Model file for the job. Use its own axes, mm. A direction names the side the tool comes from. Round coordinates to 2 decimals unless told otherwise and drop trailing zeros. Order: outer loops, then holes, each group sorted by start corner. A loop starts at its lowest first (then second) coordinate and runs counter-clockwise, first axis right, second up. Notation, with made-up numbers: (81.25, 52.5) -> (120.25, 52.5) arc R29 ccw to (120.25, 91.5) -> close; hole circle Ø9 at (25.5, 11.5). An arc over 180 degrees is marked (long way). Use CSV: the item, a comma, the result in double quotes.
```python
from build123d import *

# Parameters (mm, degrees)
PAD002_DEPTH             = 2.7
CYLINDER_R               = 2.95
CYLINDER_DEPTH           = 7
CYLINDER001_R            = 1.7
CYLINDER001_DEPTH        = 30
CLONE118_PLACEMENT_ANGLE = 180
BOX250_W                 = 10
BOX250_H                 = 10
BOX250_DEPTH             = 20


with BuildPart() as clone_of_m3nuthousing009:
    # Sketch003 → Pad002 (new body)
    with BuildSketch(Plane.XY):
        Polygon((0, 0), (1.674316, 2.9), (21.674316, 2.9), (21.674316, -2.9), (1.674316, -2.9), align=None)
    extrude(amount=PAD002_DEPTH)


with BuildPart() as clone_of_m3nuthousing009_1:
    # Clone119 placement: moved
    add(clone_of_m3nuthousing009.part.moved(Location((1.5, 5, 14))))


with BuildPart() as m3bolthead:
    # Cylinder → Cylinder (new body)
    with BuildSketch(Plane.XY):
        Circle(CYLINDER_R)
    extrude(amount=CYLINDER_DEPTH)


with BuildPart() as fusion051:
    # Cylinder001 → Cylinder001 (new body)
    with BuildSketch(Plane.XY.offset(6)):
        Circle(CYLINDER001_R)
    extrude(amount=CYLINDER001_DEPTH)

    # Fusion: union M3BoltHead
    add(m3bolthead.part)


with BuildPart() as fusion051_1:
    # Clone118 placement: moved
    add(fusion051.part.moved(Location((5, 5, 40))).rotate(Axis((5, 5, 40), (1, 0, 0)), CLONE118_PLACEMENT_ANGLE))

    # Fusion051: union Clone of M3NutHousing009
    add(clone_of_m3nuthousing009_1.part)


with BuildPart() as obj1:
    # Box250 → Box250 (new body)
    with BuildSketch(Plane.XY):
        with Locations((5, 5)):
            Rectangle(BOX250_W, BOX250_H)
    extrude(amount=BOX250_DEPTH)

    # Cut040: cut Fusion051
    add(fusion051_1.part, mode=Mode.SUBTRACT)


solid = obj1.part
```
Q1. Pin check, flat tip, straight feed: pin 1 (3 mm diameter, centred on x = 5, y = 5, fed in from +Z). Stop position of the tip, or through.
From the geometry:
pin 1,"stops at z = 4"
Q2. Mould opens along Y. For faces 1 (the cylindrical face through (4.63, 6.66, 18.37)), 2 (the flat face through (5, 10, 10)), 3 (the flat face through (5, 5, 0)) say: +Y half, -Y half, draft (parallel to the pull), parting line (faces both ways), or undercut.
From the geometry:
face 1,"undercut"
face 2,"+Y half"
face 3,"draft"
Q3. Cut at A-A (z = 18). Give the cut face in (x, y).
From the geometry:
outline,"(0, 0) -> (10, 0) -> (10, 10) -> (0, 10) -> close; hole circle Ø3.4 at (5, 5)"
Q4. Probe line 1 along Y through (x, z) = (5.5, 16.25); line 2 along Y through (x, z) = (5, 18.2). List the from-to ranges inside material, lowest first.
From the geometry:
line 1,"y = 0 to 2.1, 7.9 to 10"
line 2,"y = 0 to 3.3, 6.7 to 10"
Q5. Cut at B-B (x = 5). Give the cut face in (y, z), plus the area to 3 significant figures.
From the geometry:
outline,"(0, 0) -> (10, 0) -> (10, 20) -> (6.7, 20) -> (6.7, 16.7) -> (7.9, 16.7) -> (7.9, 14) -> (6.7, 14) -> (6.7, 4) -> (3.3, 4) -> (3.3, 14) -> (2.1, 14) -> (2.1, 16.7) -> (3.3, 16.7) -> (3.3, 20) -> (0, 20) -> close"
area,"139 mm²"
Q6. Cut at C-C (y = 6.5). Give the cut face in (x, z).
From the geometry:
outline,"(0, 0) -> (10, 0) -> (10, 14) -> (5.8, 14) -> (5.8, 4) -> (4.2, 4) -> (4.2, 14) -> (2.37, 14) -> (2.37, 16.7) -> (4.2, 16.7) -> (4.2, 20) -> (0, 20) -> close; (5.8, 16.7) -> (10, 16.7) -> (10, 20) -> (5.8, 20) -> close"
Q7. Which spindle directions (+Z, -Z, +X, -X, +Y, -Y) get a long thin tool onto all of the face, cutting with end or side? Do faces 4 (the flat face through (5, 5, 4)), 5 (the flat face through (10, 5, 10)), 6 (the flat face through (7, 5, 14)). Say none if no direction does.
From the geometry:
face 4,"+Z"
face 5,"+Z, -Z, +X, +Y, -Y"
face 6,"+X"
Q8. Cut at D-D (x = 7). Give the cut face in (y, z), plus the area to 3 significant figures.
From the geometry:
outline,"(0, 0) -> (10, 0) -> (10, 20) -> (0, 20) -> close; hole (2.1, 14) -> (7.9, 14) -> (7.9, 16.7) -> (2.1, 16.7) -> close"
area,"184 mm²"
